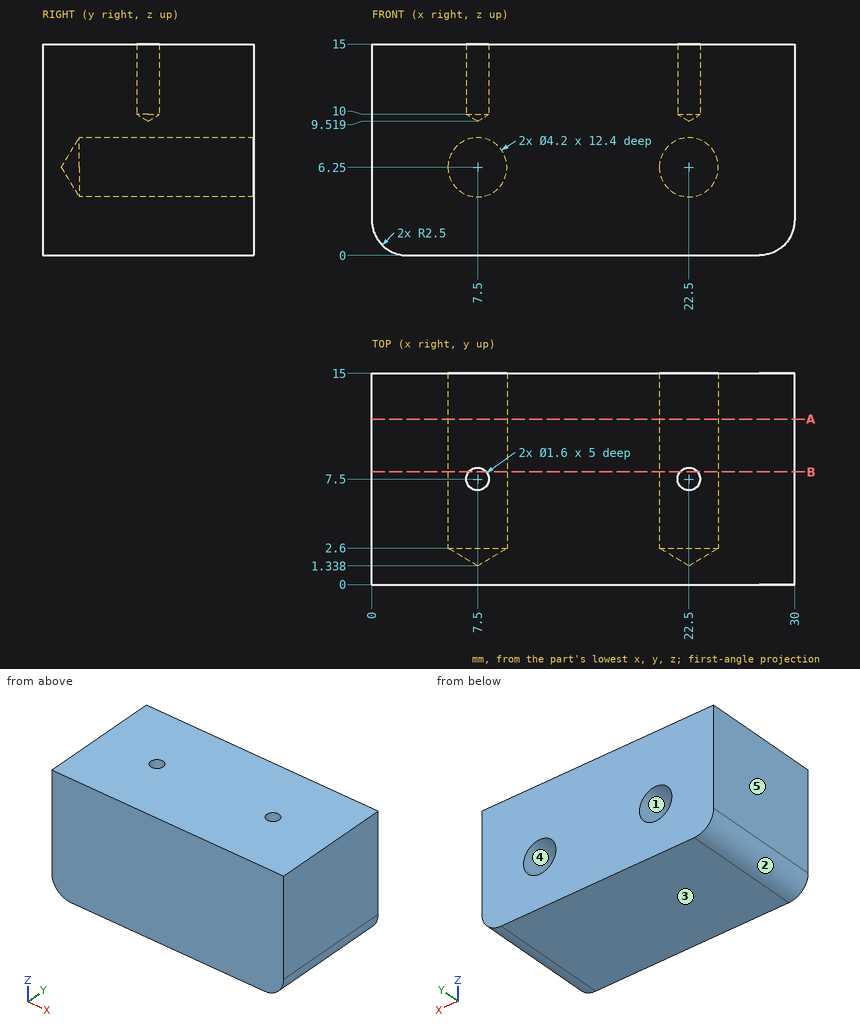
Can you work these out from the drawing? Everything is in mm from the part's minimum corner. A direction names the side the tool comes from. Coordinates: 2 decimals unless noted, no trailing zeros. Order: outer loops, then holes, each group sorted by start corner. A loop starts at its lowest first (then second) coordinate and runs counter-clockwise, first axis right, second up. Notation, with made-up numbers: (88, -17) -> (147, -17) arc R7 ccw to (147, -9) -> close; hole circle Ø9 at (-26.75, 50.25). An arc over 180 degrees is marked (long way). Return JSON: item names as keys, results as strings.
1) On a 3-axis mill with a long thin cutter (end or side, diameter ignored), from which of +Z, -Z, +X, -X, +Y, -Y can I reach the whole of each face in a straight line? I mean the marked faces 1 and 2. Say none if no direction works.
Conclusion:
{"face 1": "+Y", "face 2": "-Z, -X, +Y, -Y"}
2) I'm going to push a flat-ended pin straight in: P1, Ø1, axis at y = 8, z = 13.5, coming from the -X side. Where does the tip first touch, or does it pass through?
Conclusion:
{"P1": "stops at x = 0"}
3) Thinking about a two-plate mould opening in Z: for the marked faces 3, 4 and 5, which applies, +Z half, -Z half, draft (parallel to the pull), parting line (faces both ways), or undercut?
Conclusion:
{"face 3": "-Z half", "face 4": "undercut", "face 5": "draft"}
4) If we section it at A-A on y = 11.75: List the corners of the cut face in (x, z) for me.
Conclusion:
{"outline": "(0, 2.5) arc R2.5 ccw to (2.5, 0) -> (27.5, 0) arc R2.5 ccw to (30, 2.5) -> (30, 15) -> (0, 15) -> close; hole circle Ø4.2 at (7.5, 6.25); hole circle Ø4.2 at (22.5, 6.25)"}
5) If we section it at B-B on y = 8: State how many separate pieces and enclosed holes the cut face has, plus the area to 3 significant figures.
Conclusion:
{"separate pieces": "1", "enclosed holes": "2", "area": "407 mm²"}
6) If I drill on probe 1 along X at (y, z) = (4.75, 6.25); probe 2 along X at (y, z) = (7.5, 11.75); probe 3 along Y at (x, z) = (7.5, 13.25), over which ranges is the centre line in solid material (lowest first)?
Conclusion:
{"probe 1": "x = 0 to 5.4, 9.6 to 20.4, 24.6 to 30", "probe 2": "x = 0 to 6.7, 8.3 to 21.7, 23.3 to 30", "probe 3": "y = 0 to 6.7, 8.3 to 15"}
